Could you check a few things on this model? Use its own coordinates, in mm. A direction names the side the tool comes from. Give positions to 0.01 mm unless a question says otherwise; leave off trailing zeros. Loops run counter-clockwise (first coordinate to the right, second up) from the corner with the lowest first, then second, coordinate; pieces in that order, holes last. Notation, with made-up numbers: M -3.5,-5 L 13.5,-5 A16 cw 13.5,20 Z; hole C 60.5,85 d8. An arc over 180 degrees is marked long. Return JSON: item names as keys, results as strings. Group by question number.
1. For faces 4 (the cylindrical face through (6.634, 2.606, -1.763)), 5 (the flat face through (7, -5.54, 6)), 6 (the cylindrical face through (2.849, 4.275, -4.535)), which set-ups out of +Z, -Z, +X, -X, +Y, -Y let a thin tool reach every point of the face, with its end or its side?
2. If we section it at A-A (y = -2): Write out the boundary of the cut face in (x, z).
3. Please list where these lines run through material, in increasing order: line 1 (Z direction, x = 4.5, y = -2.5); line 2 (X direction, y = 1.5, z = 0); line 3 (Z direction, x = 3.25, y = 1.5).
4. If we mould it in two halves opening along Y, with no side actions, what happens to faces 1 (the flat face through (5.62, 4, -6)), 2 (the flat face through (4, 0, -7.938)), 3 (the flat face through (2, -6.35, 0))? For each: +Y half, -Y half, draft (parallel to the pull), parting line (faces both ways), or undercut.
5. If we section it at C-C (z = 3.75): Write out the boundary of the cut face in (x, y), plus the area to 3 significant figures.
6. If we section it at B-B (x = 5.25): Write out the boundary of the cut face in (y, z), plus the area to 3 significant figures.
7. For pin 1 (5.5 mm diameter, centred on y = -2.54, z = 4.76, fed in from -X); pin 2 (3 mm diameter, centred on y = 2.54, z = -4.76, fed in from -X); pin 3 (3 mm diameter, centred on y = 2, z = -5, fed in from +X), each with a flat end and sliding along its axis, tell me the tip position at first contact or that it passes through.
8. If we section it at D-D (z = -6.75): Write out the boundary of the cut face in (x, y).
```python
from build123d import *

# Parameters (mm, degrees)
SKETCH1_W           = 12.7
SKETCH1_H           = 15.875
BOSS_EXTRUDE1_DEPTH = 7.62
SKETCH3_R           = 1.75
CUT_EXTRUDE1_DEPTH  = 22.2885
SKETCH4_R           = 1.75
CUT_EXTRUDE2_DEPTH  = 22.2885
SKETCH5_R           = 3
SKETCH5_R_2         = 1.75
CUT_EXTRUDE3_DEPTH  = 2


with BuildPart() as part:
    # Sketch1 → Boss-Extrude1 (new body)
    with BuildSketch(Plane.YZ):
        Rectangle(SKETCH1_W, SKETCH1_H)
    extrude(amount=BOSS_EXTRUDE1_DEPTH)

    # Sketch3 → Cut-Extrude1 (cut)
    with BuildSketch(Plane.XZ.offset(6.35)):
        with Locations(Location((4.36625, 0, 0), (0, 0, 270))):
            Circle(SKETCH3_R)
    extrude(amount=-CUT_EXTRUDE1_DEPTH, mode=Mode.SUBTRACT)

    # Sketch4 → Cut-Extrude2 (cut)
    with BuildSketch(Plane.YZ.offset(7.62)):
        with Locations(Location((-2.54, 4.7625, 0), (0, 0, 270))):
            Circle(SKETCH4_R)
        with Locations(Location((2.54, -4.7625, 0), (0, 0, 270))):
            Circle(SKETCH4_R)
    extrude(amount=-CUT_EXTRUDE2_DEPTH, mode=Mode.SUBTRACT)

    # Sketch5 → Cut-Extrude3 (cut)
    # profile 1 of 4: a face of its own
    with BuildSketch(Plane.YZ.offset(7.62)):
        with Locations((-2.54, 4.7625)):
            Circle(SKETCH5_R)
        with Locations(Location((-2.54, 4.7625, 0), (0, 0, 270))):
            Circle(SKETCH5_R_2, mode=Mode.SUBTRACT)
    # profile 2 of 4: a face of its own
    with BuildSketch(Plane.YZ.offset(7.62)):
        with BuildLine():
            Line((-5.54, 7.9375), (-5.54, 4.7625))
            ThreePointArc((-5.54, 4.7625), (-2.54, 7.7625), (0.46, 4.7625))
            Line((0.46, 4.7625), (0.46, 7.9375))
            Line((0.46, 7.9375), (-5.54, 7.9375))
        make_face()
    # profile 3 of 4: a face of its own
    with BuildSketch(Plane.YZ.offset(7.62)):
        with Locations((2.54, -4.7625)):
            Circle(SKETCH5_R)
        with Locations(Location((2.54, -4.7625, 0), (0, 0, 270))):
            Circle(SKETCH5_R_2, mode=Mode.SUBTRACT)
    # profile 4 of 4: a face of its own
    with BuildSketch(Plane.YZ.offset(7.62)):
        with BuildLine():
            Line((5.54, -7.9375), (5.54, -4.7625))
            ThreePointArc((5.54, -4.7625), (2.54, -7.7625), (-0.46, -4.7625))
            Line((-0.46, -4.7625), (-0.46, -7.9375))
            Line((-0.46, -7.9375), (5.54, -7.9375))
        make_face()
    extrude(amount=-CUT_EXTRUDE3_DEPTH, mode=Mode.SUBTRACT)


solid = part.part
```
Answer:
{
 "1": {"face 4": "-Z, +X", "face 5": "+Z, +X", "face 6": "+X, -X"},
 "2": {"outline": "M 0,-7.94 L 7.62,-7.94 L 7.62,1.81 L 5.62,1.81 L 5.62,3.1 L 0,3.1 Z; M 0,6.43 L 5.62,6.43 L 5.62,7.94 L 0,7.94 Z; hole C 4.37,0 d3.5"},
 "3": {"line 1": "z = -7.94 to -1.74, 1.74 to 3.01, 6.51 to 7.94", "line 2": "x = 0 to 2.62, 6.12 to 7.62", "line 3": "z = -7.94 to -6.17, -3.36 to -1.35, 1.35 to 7.94"},
 "4": {"face 1": "undercut", "face 2": "draft", "face 3": "-Y half"},
 "5": {"outline": "M 0,-6.35 L 7.62,-6.35 L 7.62,-5.36 L 5.62,-5.36 L 5.62,-3.97 L 0,-3.97 Z; M 0,-1.11 L 5.62,-1.11 L 5.62,0.28 L 7.62,0.28 L 7.62,6.35 L 0,6.35 Z", "area": "69.4 mm²"},
 "6": {"outline": "M -6.35,-7.94 L 6.35,-7.94 L 6.35,-1.51 L -6.35,-1.51 Z; M -6.35,1.51 L 6.35,1.51 L 6.35,7.94 L -6.35,7.94 Z; hole C -2.54,4.76 d3.5; hole C 2.54,-4.76 d3.5", "area": "144 mm²"},
 "7": {"pin 1": "stops at x = 0", "pin 2": "passes through", "pin 3": "stops at x = 5.62"},
 "8": {"outline": "M 0,-6.35 L 7.62,-6.35 L 7.62,-0.46 L 5.62,-0.46 L 5.62,5.54 L 7.62,5.54 L 7.62,6.35 L 0,6.35 Z"}
}
